Can you work these out from the drawing? Everything is in mm from the part's minimum corner. Give positions to 0.01 mm unless a question says otherwise; leave off trailing zeros. Loops run counter-clockwise (first coordinate to the right, second up) from the corner with the lowest first, then second, coordinate; pieces in that order, holes last. Notation, with made-up numbers: (51, -21.5) - (90, -21.5) arc R12 cw to (90, -14.5) - close; hole circle Ø1 at (68.5, 5.25). An arc over 180 degrees is marked (long way). One line per item, written item: value. Start each with the question number.
Q1. I'm going to push a flat-ended pin straight in: P1, Ø1, axis at x = 3.5, z = 53, coming from the -Y side. Where does the tip first touch, or does it pass through?
Q2. I want a section at B-B (z = 13). Please give me the cut outline in (x, y).
Q3. If I drill on line 1 (Z direction, x = 3, y = 0.5); line 2 (X direction, y = 3.25, z = 94.5), over which ranges is the centre line in solid material (lowest first)? Write a range as from..to.
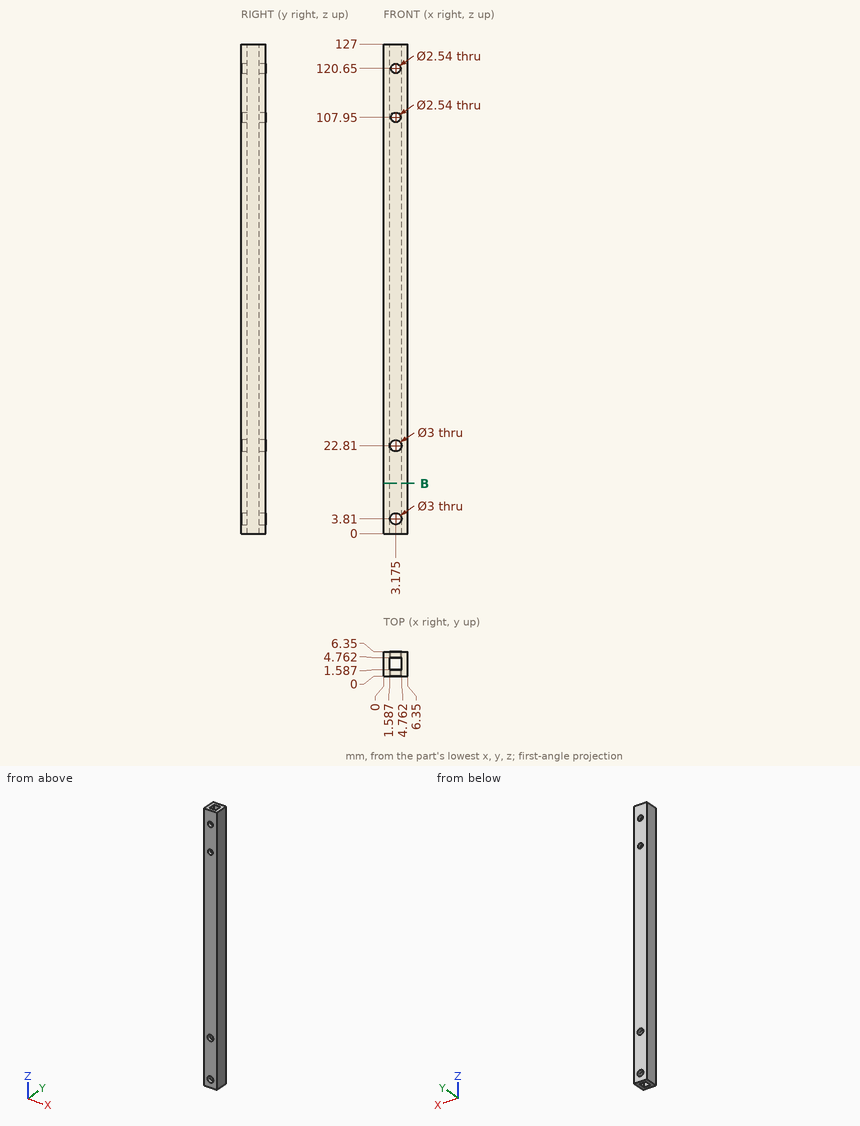
Worked answers:
1. P1: stops at y = 0
2. outline: (0, 0) - (6.35, 0) - (6.35, 6.35) - (0, 6.35) - close; hole (1.59, 1.59) - (4.76, 1.59) - (4.76, 4.76) - (1.59, 4.76) - close
3. line 1: z = 0..2.32, 5.3..21.32, 24.3..106.69, 109.21..119.39, 121.91..127
3. line 2: x = 0..1.59, 4.76..6.35
